Answer from the drawing. Dimensions are ordinates in mm from the lowest x, y and z of the part. Round coordinates to 2 decimals unless told otherwise and drop trailing zeros. Write each loop counter-clockwise with the first axis right and the second up, starting at its lowest first coordinate (ties: lowest second). Pieces come first, ordered by that corner, then holes.
1. Straight lines are drawn through the part: probe 1 along Z at (x, y) = (77.4, 1); probe 2 along X at (y, z) = (1.15, 69.9); probe 3 along Z at (x, y) = (124.2, 1.15). For each, find the intervals that lie inside material, in ascending order.
2. Find section A-A (y = 0.8). Write down the section's boundary in (x, z), and give its area (3 significant figures).
3. Find section B-B (x = 77.4). Write down the section's boundary in (y, z), and give its area (3 significant figures).
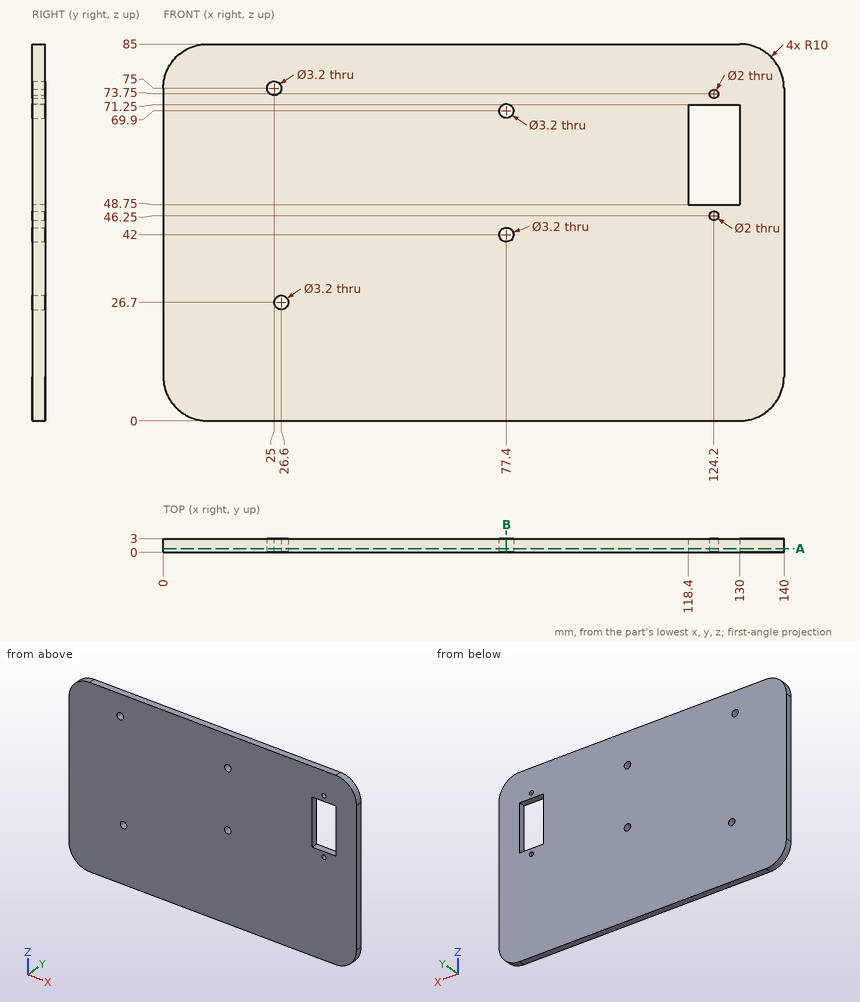
Worked answers:
1. probe 1: z = 0 to 40.4, 43.6 to 68.3, 71.5 to 85
1. probe 2: x = 0 to 75.8, 79 to 118.4, 130 to 140
1. probe 3: z = 0 to 45.25, 47.25 to 48.75, 71.25 to 72.75, 74.75 to 85
2. outline: (0, 10) arc R10 ccw to (10, 0) - (130, 0) arc R10 ccw to (140, 10) - (140, 75) arc R10 ccw to (130, 85) - (10, 85) arc R10 ccw to (0, 75) - close; hole circle Ø3.2 at (25, 75); hole circle Ø3.2 at (26.6, 26.7); hole circle Ø3.2 at (77.4, 42); hole circle Ø3.2 at (77.4, 69.9); hole (118.4, 48.75) - (130, 48.75) - (130, 71.25) - (118.4, 71.25) - close; hole circle Ø2 at (124.2, 46.25); hole circle Ø2 at (124.2, 73.75)
2. area: 11,500 mm2
3. outline: (0, 0) - (3, 0) - (3, 40.4) - (0, 40.4) - close; (0, 43.6) - (3, 43.6) - (3, 68.3) - (0, 68.3) - close; (0, 71.5) - (3, 71.5) - (3, 85) - (0, 85) - close
3. area: 236 mm2
